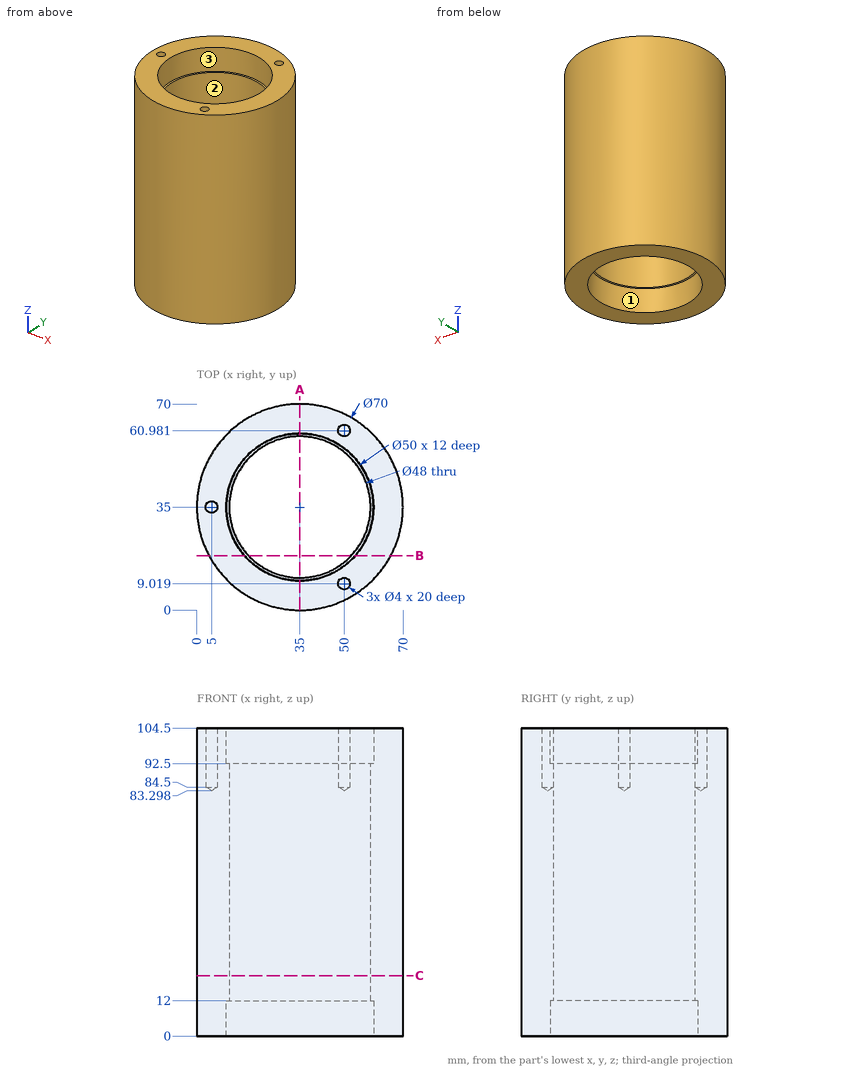
Here's the drawing with two shaded views (mm, measured from the low corner). I have some questions. A direction names the side the tool comes from. Round coordinates to 2 decimals unless told otherwise and drop trailing zeros. Write each loop counter-clockwise with the first axis right and the second up, starting at its lowest first coordinate (ties: lowest second). Pieces come first, ordered by that corner, then holes. Notation, with made-up numbers: M -10,-21.5 L 9,-21.5 A25 cw 9,11.5 Z; hole C -5,-29.5 d11. An arc over 180 degrees is marked long. Answer in a Markdown table with one row per item. Add a question column.
Q1. Imagine slicing it at C-C (z = 20.5). Please give me the cut outline in (x, y), then the cut area to 3 significant figures.
Q2. On a 3-axis mill with a long thin cutter (end or side, diameter ignored), from which of +Z, -Z, +X, -X, +Y, -Y can I reach the whole of each face in a straight line? I mean the marked faces 1, 2 and 3. Say none if no direction works.
Q3. Imagine slicing it at A-A (x = 35). Please give me the cut outline in (y, z), then the cut area to 3 significant figures.
Q4. If I drill on line 1 (X direction, y = 35.5, z = 70) (1 decimal); line 2 (Y direction, x = 50, z = 89.5) (1 decimal); line 3 (X direction, y = 31, z = 84.5) (1 decimal), over which ranges is the centre line in solid material (lowest first)? Write a range as from..to.
Q5. Imagine slicing it at B-B (y = 18.5). Please give me the cut outline in (x, z), then the cut area to 3 significant figures.
Q6. Will these pins go through, and if not, where does the flat tip stop? pin 1 Ø1.5 at (y, z) = (18.5, 69.5) entering from -X; pin 2 Ø2.5 at (x, y) = (5, 35) entering from +Z; pin 3 Ø5 at (x, y) = (40, 14) entering from +Z.
Values:
| question | item | result |
|---|---|---|
| 1 | outline | C 35,35 d70; hole C 35,35 d48 |
| 1 | area | 2,040 mm^2 |
| 2 | face 1 | -Z |
| 2 | face 2 | +Z, -Z |
| 2 | face 3 | +Z |
| 3 | outline | M 0,0 L 10,0 L 10,12 L 11,12 L 11,92.5 L 10,92.5 L 10,104.5 L 0,104.5 Z; M 59,12 L 60,12 L 60,0 L 70,0 L 70,104.5 L 60,104.5 L 60,92.5 L 59,92.5 Z |
| 3 | area | 2,250 mm^2 |
| 4 | line 1 | 0..11, 59..70 |
| 4 | line 2 | 3.4..7, 11..16.3, 53.7..59, 63..66.6 |
| 4 | line 3 | 0.2..11.3, 58.7..69.8 |
| 5 | outline | M 4.13,0 L 16.22,0 L 16.22,12 L 17.57,12 L 17.57,92.5 L 16.22,92.5 L 16.22,104.5 L 4.13,104.5 Z; M 52.43,12 L 53.78,12 L 53.78,0 L 65.87,0 L 65.87,104.5 L 53.78,104.5 L 53.78,92.5 L 52.43,92.5 Z |
| 5 | area | 2,740 mm^2 |
| 6 | pin 1 | x = 3.74 |
| 6 | pin 2 | z = 84.05 |
| 6 | pin 3 | z = 92.5 |
